Can you work these out from the model? Positions are in its coordinate system, mm. A direction names the side the tool comes from. Give positions to 0.01 mm unless a question says otherwise; leave off trailing zeros. Loops run counter-clockwise (first coordinate to the right, second up) from the corner with the lowest first, then second, coordinate; pieces in that order, holes last. Notation, with made-up numbers: (53, 5.5) -> (93, 5.5) arc R33 cw to (93, 38.5) -> close; hole circle Ø10 at (34.5, -21.75). An arc over 180 degrees is marked (long way). Use CSV: the item, a comma, the result in double quotes.
from build123d import *

# Parameters (mm, degrees)
F1_DEPTH  = 57.15
F3_DEPTH  = 5.08
F5_DEPTH  = 41.402
F7_DEPTH  = 53.975
F8_W      = 41.1952470895
F8_H      = 60.1872038096
F9_DEPTH  = 25.4
F11_DEPTH = 114.3
F12_W     = 114.3
F12_H     = 56.9759604018
F13_DEPTH = 12.7
F15_DEPTH = 114.3
F17_DEPTH = 8.89
F18_R     = 19.3940377175
F19_DEPTH = 8.89


with BuildPart() as f1:
    # F0 (on Right) → F1 (new body, symmetric)
    with BuildSketch(Plane.YZ):
        with BuildLine():
            Line((-92.7504450083, 16.9447939843), (-92.7504450083, -46.5026274323))
            Line((-92.7504450083, -46.5026274323), (134.5391124487, -46.5026274323))
            Line((134.5391124487, -46.5026274323), (134.5391124487, 24.8438697308))
            ThreePointArc((134.5391124487, 24.8438697308), (116.7467916318, 53.6046661319), (84.8513692617, 64.848870039))
            Line((84.8513692617, 64.848870039), (-44.8463708162, 64.848870039))
            Line((-44.8463708162, 64.848870039), (-92.7504450083, 16.9447939843))
        make_face()
    extrude(amount=F1_DEPTH, both=True)

    # F2 (on face) → F3 (join)
    with BuildSketch(Plane(origin=(0, 0, -46.5026274323), x_dir=(1, 0, 0), z_dir=(0, 0, -1))):
        Polygon((-28.575, -77.7167230844), (0, -134.5391124487), (28.575, -77.7167230844), (57.15, -20.8943337202), (-57.15, -20.8943337202), align=None)
        Polygon((28.575, -77.7167230844), (0, -134.5391124487), (8.5433015109, -134.5391124487), align=None)
        Polygon((-8.5433015109, -134.5391124487), (0, -134.5391124487), (-28.575, -77.7167230844), align=None)
        Polygon((8.5433015109, -134.5391124487), (0, -134.5391124487), (-8.5433015109, -134.5391124487), (0, -158.7732434273), align=None)
    extrude(amount=-F3_DEPTH)

    # F4 (on face) → F5 (cut)
    with BuildSketch(Plane(origin=(0, 0, -46.5026274323), x_dir=(1, 0, 0), z_dir=(0, 0, -1))):
        Polygon((-4.6747997403, -134.5391124487), (0, -146.656177938), (4.2716507554, -134.5391124487), align=None)
    extrude(amount=-F5_DEPTH, mode=Mode.SUBTRACT)

    # F6 (on Right) → F7 (cut, symmetric)
    with BuildSketch(Plane.YZ):
        with BuildLine():
            Line((-89.0294536948, 15.1805384085), (-89.0294536948, -41.0569272935))
            Line((-89.0294536948, -41.0569272935), (130.7652890682, -41.0569272935))
            Line((130.7652890682, -41.0569272935), (130.7652890682, 25.959385559))
            ThreePointArc((130.7652890682, 25.959385559), (115.7413511895, 50.5424798047), (88.5871946812, 60.1705126464))
            Line((88.5871946812, 60.1705126464), (-44.0394952893, 60.1705126464))
            Line((-44.0394952893, 60.1705126464), (-89.0294536948, 15.1805384085))
        make_face()
    extrude(amount=F7_DEPTH, both=True, mode=Mode.SUBTRACT)

    # F8 (on face) → F9 (cut, symmetric)
    with BuildSketch(Plane.YZ.offset(57.15)):
        with Locations((-24.2487472715, -13.1488079205)):
            Rectangle(F8_W, F8_H)
    extrude(amount=F9_DEPTH, both=True, mode=Mode.SUBTRACT)

    # F10 (on face) → F11 (join)
    with BuildSketch(Plane.YZ.offset(57.15)):
        Polygon((-92.7504450083, -11.7301335558), (-92.7504450083, -14.778916724), (-47.2835078835, -14.778916724), (-47.2835078835, -11.7301335558), (-63.0396455526, -11.7301335558), (-63.0396455526, 16.9447939843), (-47.2835078835, 16.9447939843), (-47.2835078835, 62.4117328769), (-49.9636399546, 59.7316007017), (-49.9636399546, 20.691152662), (-65.4636770487, 20.691152662), (-65.4636770487, -11.7301335558), align=None)
    extrude(amount=-F11_DEPTH)

    # F12 (on face) → F13 (cut)
    with BuildSketch(Plane(origin=(0, -54.8476212995, 54.8476191669), x_dir=(1, 0, 0), z_dir=(0, -0.7071067949, 0.7071067674))):
        with Locations((0, -25.1147081824)):
            Rectangle(F12_W, F12_H)
    extrude(amount=-F13_DEPTH, mode=Mode.SUBTRACT)

    # F14 (on face) → F15 (cut)
    with BuildSketch(Plane.YZ.offset(57.15)):
        Polygon((-92.7504450083, 16.9447939843), (-92.7504450083, 6.4976271242), (-78.9771229029, 6.4976271242), (-78.9771229029, 12.7576040339), (-83.7701887126, 7.9645380378), align=None)
    extrude(amount=-F15_DEPTH, mode=Mode.SUBTRACT)

    # F16 (on face) → F17 (join)
    with BuildSketch(Plane.YZ.offset(57.15)):
        with BuildLine():
            Line((20.8943337202, -46.5026274323), (40.6107781849, -46.5026274323))
            ThreePointArc((40.6107781849, -46.5026274323), (20.8943337202, -26.7861829676), (1.1778892555, -46.5026274323))
            Line((1.1778892555, -46.5026274323), (20.8943337202, -46.5026274323))
        make_face()
        with BuildLine():
            ThreePointArc((1.1778892555, -46.5026274323), (20.8943337202, -66.2190718971), (40.6107781849, -46.5026274323))
            Line((40.6107781849, -46.5026274323), (20.8943337202, -46.5026274323))
            Line((20.8943337202, -46.5026274323), (1.1778892555, -46.5026274323))
        make_face()
    extrude(amount=F17_DEPTH)

    # F18 (on face) → F19 (join)
    with BuildSketch(Plane(origin=(-57.15, 0, 0), x_dir=(0, -1, 0), z_dir=(-1, 0, 0))):
        with Locations((-20.8943337202, -46.5026274323)):
            Circle(F18_R)
    extrude(amount=F19_DEPTH)


solid = f1.part
(1) We'd pull the mould along Y, two halves only. Please class faces 5 (the face through (-61.533, 2.396, -40.677)), 6 (the face through (1, -92.75, -20)), 7 (the face through (1, 23, 60.171)), 8 (the face through (1, 21, 64.849)): released by +Y, released by -Y, zero draft, split by the parting line, or undercut.
Answer sheet:
face 5,"split by the parting line"
face 6,"released by -Y"
face 7,"undercut"
face 8,"zero draft"
(2) If we section it at C-C, the plane y = -14: Write out the boundary of the cut face in (x, z) (3 decimals), then the cut area to 3 significant figures.
Answer sheet:
outline,"(-57.15, -46.503) -> (57.15, -46.503) -> (57.15, -43.242) -> (31.75, -43.242) -> (31.75, -41.057) -> (-53.975, -41.057) -> (-53.975, 60.171) -> (53.975, 60.171) -> (53.975, 16.945) -> (57.15, 16.945) -> (57.15, 64.849) -> (-57.15, 64.849) -> close"
area,"1,560 mm2"
(3) Will these pins go through, and if not, where does the flat tip stop? pin 1 Ø8 at (x, z) = (-43, 20) entering from +Y; pin 2 Ø1 at (x, z) = (48, 28) entering from -Y; pin 3 Ø5 at (x, z) = (6.5, 47) entering from +Y.
Answer sheet:
pin 1,"stops at y = 134.54"
pin 2,"stops at y = -49.96"
pin 3,"stops at y = 125.54"
(4) If we section it at A-A, the plane z = 2: Write out the boundary of the cut face in (x, y) (3 decimals), then the cut area to 3 significant figures.
Answer sheet:
outline,"(-57.15, -92.75) -> (57.15, -92.75) -> (57.15, -44.846) -> (53.975, -44.846) -> (53.975, -63.04) -> (-53.975, -63.04) -> (-53.975, 130.765) -> (53.975, 130.765) -> (53.975, -3.651) -> (57.15, -3.651) -> (57.15, 134.539) -> (-57.15, 134.539) -> close; hole (-53.975, -89.029) -> (53.975, -89.029) -> (53.975, -65.464) -> (-53.975, -65.464) -> close"
area,"2,380 mm2"
(5) If I drill on L1, parallel to Y at x = -53.5, z = 20; L2, parallel to X at y = -13.5, z = 40.5 (3 decimals); L3, parallel to Y at x = -13, z = -26.5, over which ranges is the centre line in solid material (lowest first)? Write a range as from..to.
Answer sheet:
L1,"y = -65.46..-47.28, 130.77..134.54"
L2,"x = -57.15..-53.975, 53.975..57.15"
L3,"y = -92.75..-89.03, 130.77..134.54"
(6) If we section it at B-B, the plane x = -37.5: Write out the boundary of the cut face in (y, z).
Answer sheet:
outline,"(-92.75, -46.5) -> (134.54, -46.5) -> (134.54, 24.84) arc R50.86 ccw to (84.85, 64.85) -> (-44.85, 64.85) -> (-52.46, 57.23) -> (-47.28, 52.05) -> (-47.28, 56.93) -> (-44.04, 60.17) -> (88.59, 60.17) arc R43.11 cw to (130.77, 25.96) -> (130.77, -41.06) -> (-89.03, -41.06) -> (-89.03, -14.78) -> (-47.28, -14.78) -> (-47.28, -11.73) -> (-63.04, -11.73) -> (-63.04, 16.94) -> (-47.28, 16.94) -> (-47.28, 44.45) -> (-49.96, 41.77) -> (-49.96, 20.69) -> (-65.46, 20.69) -> (-65.46, -11.73) -> (-89.03, -11.73) -> (-89.03, 6.5) -> (-92.75, 6.5) -> close"
(7) If we section it at D-D, the plane z = -37.5: Write out the boundary of the cut face in (x, y) (3 decimals), then the cut area to 3 significant figures.
Answer sheet:
outline,"(-66.04, 3.716) -> (-57.15, 3.716) -> (-57.15, -92.75) -> (57.15, -92.75) -> (57.15, -44.846) -> (53.975, -44.846) -> (53.975, -89.029) -> (-53.975, -89.029) -> (-53.975, 130.765) -> (53.975, 130.765) -> (53.975, -3.651) -> (57.15, -3.651) -> (57.15, 3.353) -> (66.04, 3.353) -> (66.04, 38.435) -> (57.15, 38.435) -> (57.15, 134.539) -> (-57.15, 134.539) -> (-57.15, 38.072) -> (-66.04, 38.072) -> close"
area,"2,740 mm2"
(8) Which directions (+Z, -Z, +X, -X, +Y, -Y) give clear straight access to the entire face, cutting with the end or side of a thin tool? Please do faces 1 (the face through (45, -25, -43.242)), 2 (the face through (1, -89.029, -28)), 3 (the face through (1, -49.964, 31)), 4 (the face through (-0.8, -50.03, 54.8)).
Answer sheet:
face 1,"+X"
face 2,"none"
face 3,"-Y"
face 4,"+X, -X, -Y"
